The model under review builds one solid part; all positions refer to its coordinate system, in mm. A direction names the side the tool comes from. Coordinates: 2 decimals unless noted, no trailing zeros. Use one line per item in the form item = value. Start each with the question number.
(1) Mouldability with a two-part tool opening along Z and no side actions: class faces 3 (the flat face through (4, 10, 2.56)), 4 (the flat face through (-250, 0, 0)), 5 (the flat face through (-3, 0, 9.95)), 6 (the flat face through (4, -10, -2.56)) as +Z half, -Z half, draft (parallel to the pull), parting line (faces both ways), or undercut.
(2) Wall thickness on line 1 along Y through (x, z) = (-196, -6); line 2 along Z through (x, y) = (121, -14.5); line 3 along Z through (x, y) = (-27.5, -12): over which ranges is each line inside the solid? List them lowest first.
(3) For faces 1 (the flat face through (-3, 19.91, 0)), 2 (the flat face through (4, 10, -2.56)), list the 3-axis set-ups (+Z, -Z, +X, -X, +Y, -Y) from which the entire face can be reached by the end or side of a thin tool; tool diameter is ignored.
```python
from build123d import *

# Parameters (mm, degrees)
SKETCH1_W            = 500
SKETCH1_H            = 19.9
BOSS_EXTRUDE1_DEPTH  = 19.91
CUT_EXTRUDE1_DEPTH   = 501.495165411
MIRROR2_COPY_1_DEPTH = 501.495165411


with BuildPart() as part:
    # Sketch1 → Boss-Extrude1 (new, symmetric)
    with BuildSketch(Plane(origin=(0, 0, 0), x_dir=(1, 0, 0), z_dir=(0, 1, 0))):
        Rectangle(SKETCH1_W, SKETCH1_H)
    extrude(amount=BOSS_EXTRUDE1_DEPTH, both=True)

    # Sketch2 → Cut-Extrude1 (cut, through all)
    with BuildSketch(Plane(origin=(250, 0, 0), x_dir=(0, 0, -1), z_dir=(1, 0, 0))):
        Polygon((-9.95, 7.42), (-8.45, 7.42), (-8.45, 4.92), (-2.56, 4.92), (-2.56, 15.09), (-8.45, 15.09), (-8.45, 12.59), (-9.95, 12.59), align=None)
    cut_extrude1 = extrude(amount=-CUT_EXTRUDE1_DEPTH, mode=Mode.SUBTRACT)

    # Mirror1: Cut-Extrude1 across plane
    add(cut_extrude1.mirror(Plane.XY), mode=Mode.SUBTRACT)

    # Mirror2: Cut-Extrude1 across plane
    add(cut_extrude1.mirror(Plane.ZX), mode=Mode.SUBTRACT)

    # Mirror2 copy 1 sketch → Mirror2 copy 1 (cut, through all)
    with BuildSketch(Plane(origin=(250, 0, 0), x_dir=(0, 0, 1), z_dir=(1, 0, 0))):
        Polygon((-9.95, 7.42), (-8.45, 7.42), (-8.45, 4.92), (-2.56, 4.92), (-2.56, 15.09), (-8.45, 15.09), (-8.45, 12.59), (-9.95, 12.59), align=None)
    extrude(amount=-MIRROR2_COPY_1_DEPTH, mode=Mode.SUBTRACT)


solid = part.part
```
Findings:
q1.face_3 = undercut
q1.face_4 = draft
q1.face_5 = +Z half
q1.face_6 = undercut
q2.line_1 = -19.91 to -15.09, -4.92 to 4.92, 15.09 to 19.91
q2.line_2 = -9.95 to -8.45, -2.56 to 2.56, 8.45 to 9.95
q2.line_3 = -2.56 to 2.56
q3.face_1 = +Z, -Z, +X, -X, +Y
q3.face_2 = +X, -X
